For this review, take the finished solid that the model builds, in its own axes (mm). Give positions to 0.01 mm unless a question says otherwise; leave off trailing zeros. Write each loop counter-clockwise with the first axis right and the second up, starting at its lowest first coordinate (ties: lowest second). Pieces come first, ordered by that corner, then holes. Notation, with made-up numbers: (88, 44) -> (111, 44) arc R21 ccw to (111, 56) -> close; hole circle Ø1 at (61.25, 40). An arc over 180 degrees is marked (long way). Return JSON: item names as keys, results as strings.
Autodesk Inventor part; units mm, degrees
ref_plane "YZ Plane" through (0, 0, 0) normal (1, 0, 0) x (0, 1, 0)
ref_plane "XZ Plane" through (0, 0, 0) normal (0, 1, 0) x (-1, 0, 0)
ref_plane "XY Plane" through (0, 0, 0) normal (0, 0, 1) x (1, 0, 0)
sketch "Sketch1" plane through (0, 0, 0) normal (0, 1, 0) x (-1, 0, 0)
  arc A0 (-177, 0) -> (177, 0) centre (0, 0) ccw
  line L0 (-177, 0) -> (-177, 151.6)
  line L1 (-151.6, 177) -> (151.6, 177)
  line L2 (177, 151.6) -> (177, 0)
  arc A1 (-151.6, 177) -> (-177, 151.6) centre (-151.6, 151.6) ccw
  arc A2 (177, 151.6) -> (151.6, 177) centre (151.6, 151.6) ccw
  point P0 (-177, 177)
  point P1 (177, 177)
  dimension "d0" = 354
  dimension "d98" = 177
  dimension "d99" = 177
  dimension "d101" = 354
  dimension "d102" = 177
  dimension "d217" = 25.4
extrude "Extrusion1" add sketch "Sketch1" along normal blind 4.7625
sketch "Sketch8" plane through (0, 4.7625, 0) normal (0, 1, 0) x (1, 0, 0)
  circle A0 centre (101.6, -101.6) radius 1.7
  circle A1 centre (101.6, 101.6) radius 1.7
  circle A2 centre (-101.6, 101.6) radius 1.7
  circle A3 centre (-101.6, -101.6) radius 1.7
  arc A4 (177, 0) -> (-177, 0) centre (0, 0) ccw construction
  line L0 (0, 177) -> (0, -177) construction
  line L1 (-151.6, -177) -> (151.6, -177) construction
  line L2 (-177, 0) -> (-177, -151.6) construction
  line L3 (177, -151.6) -> (177, 0) construction
  line L4 (-177, 0) -> (177, 0) construction
  point P0 (0, 0)
  point P1 (-177, -177)
  point P2 (177, -177)
  dimension "d103" = 3.4
  dimension "d104" = 3.4
  dimension "d105" = 3.4
  dimension "d106" = 3.4
  dimension "d115" = 101.6
  dimension "d116" = 101.6
  dimension "d117" = 101.6
  dimension "d118" = 101.6
  dimension "d119" = 101.6
  dimension "d120" = 101.6
  dimension "d121" = 101.6
  dimension "d122" = 101.6
extrude "Stand-Offs" cut sketch "Sketch8" against normal through all
sketch "Sketch9" plane through (0, 4.7625, 0) normal (0, 1, 0) x (1, 0, 0)
  line L0 (-150.65, -79.3) -> (-150.65, -164.3)
  line L1 (-150.65, -164.3) -> (-120.65, -164.3)
  line L2 (-120.65, -164.3) -> (-120.65, -79.3)
  line L3 (-120.65, -79.3) -> (-150.65, -79.3)
  circle A0 centre (-114.3, -96.4) radius 1.7
  circle A1 centre (-114.3, -147.2) radius 1.7
  circle A2 centre (-157, -147.2) radius 1.7
  circle A3 centre (-157, -96.4) radius 1.7
  arc A4 (177, 0) -> (-177, 0) centre (0, 0) ccw construction
  line L4 (0, 177) -> (0, -177) construction
  line L5 (-151.6, -177) -> (151.6, -177) construction
  line L6 (-177, -177) -> (177, -177) construction
  line L7 (-120.65, -121.8) -> (-150.65, -121.8) construction
  line L8 (150.65, -164.3) -> (120.65, -164.3)
  line L9 (120.65, -164.3) -> (120.65, -79.3)
  line L10 (120.65, -79.3) -> (150.65, -79.3)
  circle A5 centre (114.3, -96.4) radius 1.7
  circle A6 centre (114.3, -147.2) radius 1.7
  line L11 (150.65, -79.3) -> (150.65, -164.3)
  circle A7 centre (157, -96.4) radius 1.7
  circle A8 centre (157, -147.2) radius 1.7
  line L12 (120.65, -121.8) -> (150.65, -121.8) construction
  point P0 (177.1241, 0)
  dimension "d126" = 30
  dimension "d129" = 3.4
  dimension "d130" = 3.4
  dimension "d131" = 3.4
  dimension "d132" = 3.4
  dimension "d133" = 6.35
  dimension "d134" = 6.35
  dimension "d135" = 6.35
  dimension "d136" = 6.35
  dimension "d141" = 120.65
  dimension "d142" = 12.7
  dimension "d143" = 85
  dimension "d144" = 25.4
  dimension "d145" = 25.4
  dimension "d146" = 25.4
  dimension "d147" = 25.4
extrude "Wheels" cut sketch "Sketch9" against normal through all
sketch "Sketch10" plane through (0, 4.7625, 0) normal (0, 1, 0) x (1, 0, 0)
  circle A0 centre (-72.47, -143.49) radius 1.7
  circle A1 centre (-21.59, -143.49) radius 1.7
  circle A2 centre (-72.47, -100.11) radius 1.7
  circle A3 centre (-21.59, -100.11) radius 1.7
  arc A4 (177, 0) -> (-177, 0) centre (0, 0) ccw construction
  line L0 (0, 177) -> (0, -177) construction
  line L1 (-151.6, -177) -> (151.6, -177) construction
  line L2 (177, -151.6) -> (177, 0) construction
  line L3 (-177, 0) -> (-177, -151.6) construction
  line L4 (177, 0) -> (-177, 0) construction
  line L5 (-150.65, -79.3) -> (-150.65, -164.3) construction
  line L6 (-150.65, -121.8) -> (150.65, -121.8) construction
  line L7 (150.65, -79.3) -> (150.65, -164.3) construction
  line L8 (-120.65, -79.3) -> (-120.65, -164.3) construction
  circle A5 centre (72.47, -143.49) radius 1.7
  circle A6 centre (72.47, -100.11) radius 1.7
  circle A7 centre (21.59, -143.49) radius 1.7
  circle A8 centre (21.59, -100.11) radius 1.7
  line L9 (-76.28, -96.3) -> (-17.78, -96.3) construction
  line L10 (-17.78, -96.3) -> (-17.78, -147.3) construction
  line L11 (-17.78, -147.3) -> (-76.28, -147.3) construction
  line L12 (-76.28, -147.3) -> (-76.28, -96.3) construction
  point P0 (-177, -177)
  point P1 (177, -177)
  dimension "d150" = 3.4
  dimension "d151" = 3.4
  dimension "d152" = 3.4
  dimension "d153" = 3.4
  dimension "d235" = 58.5
  dimension "d236" = 51
  dimension "d237" = 3.81
  dimension "d238" = 3.81
  dimension "d239" = 3.81
  dimension "d240" = 3.81
  dimension "d241" = 3.81
  dimension "d242" = 3.81
  dimension "d243" = 3.81
  dimension "d244" = 3.81
  dimension "d245" = 21.59
  dimension "d246" = 21.59
  dimension "d247" = 25.5
extrude "Motor Mount" cut sketch "Sketch10" against normal through all
sketch "Sketch11" plane through (0, 4.7625, 0) normal (0, 1, 0) x (1, 0, 0)
  circle A0 centre (-46.25, 39.25) radius 1.7
  circle A1 centre (46.25, 39.25) radius 1.7
  circle A2 centre (46.25, -39.25) radius 1.7
  circle A3 centre (-46.25, -39.25) radius 1.7
  line L0 (-177, 0) -> (-177, -151.6) construction
  arc A4 (177, 0) -> (-177, 0) centre (0, 0) ccw construction
  line L1 (-177, 0) -> (177, 0) construction
  line L2 (0, 177) -> (0, -177) construction
  line L3 (-151.6, -177) -> (151.6, -177) construction
  point P0 (-177, -177)
  point P1 (177, -177)
  dimension "d170" = 3.4
  dimension "d171" = 3.4
  dimension "d172" = 3.4
  dimension "d173" = 3.4
  dimension "d174" = 92.5
  dimension "d175" = 92.5
  dimension "d176" = 78.5
  dimension "d177" = 78.5
  dimension "d183" = 46.25
  dimension "d184" = 39.25
  dimension "d185" = 39.25
  dimension "d186" = 46.25
extrude "PCB" cut sketch "Sketch11" against normal through all
sketch "Sketch12" plane through (0, 4.7625, 0) normal (0, 1, 0) x (1, 0, 0)
  circle A0 centre (20, 132.55) radius 1.7
  circle A1 centre (-20, 132.55) radius 1.7
  line L0 (-177, 0) -> (-177, -151.6) construction
  arc A2 (177, 0) -> (-177, 0) centre (0, 0) ccw construction
  line L1 (-177, 0) -> (177, 0) construction
  arc A3 (177, 0) -> (-177, 0) centre (0, 0) ccw construction
  line L2 (0, 177) -> (0, -177) construction
  point P0 (-177, -177)
  dimension "d190" = 3.4
  dimension "d191" = 3.4
  dimension "d192" = 40
  dimension "d198" = 44.45
  dimension "d200" = 44.45
  dimension "d201" = 20
extrude "Ball Caster" cut sketch "Sketch12" against normal through all
sketch "Sketch13" plane through (0, 4.7625, 0) normal (0, 1, 0) x (1, 0, 0)
  line L0 (-34.925, 155.575) -> (-28.575, 155.575)
  line L1 (-28.575, 155.575) -> (-28.575, 152.4)
  line L2 (-28.575, 152.4) -> (-34.925, 152.4)
  line L3 (-34.925, 152.4) -> (-34.925, 155.575)
  line L4 (-22.225, 155.575) -> (-15.875, 155.575)
  line L5 (-15.875, 155.575) -> (-15.875, 152.4)
  line L6 (-15.875, 152.4) -> (-22.225, 152.4)
  line L7 (-22.225, 152.4) -> (-22.225, 155.575)
  line L8 (-9.525, 155.575) -> (-3.175, 155.575)
  line L9 (-3.175, 155.575) -> (-3.175, 152.4)
  line L10 (-3.175, 152.4) -> (-9.525, 152.4)
  line L11 (-9.525, 152.4) -> (-9.525, 155.575)
  line L12 (3.175, 155.575) -> (9.525, 155.575)
  line L13 (9.525, 155.575) -> (9.525, 152.4)
  line L14 (9.525, 152.4) -> (3.175, 152.4)
  line L15 (3.175, 152.4) -> (3.175, 155.575)
  line L16 (15.875, 155.575) -> (22.225, 155.575)
  line L17 (22.225, 155.575) -> (22.225, 152.4)
  line L18 (22.225, 152.4) -> (15.875, 152.4)
  line L19 (15.875, 152.4) -> (15.875, 155.575)
  line L20 (28.575, 155.575) -> (34.925, 155.575)
  line L21 (34.925, 155.575) -> (34.925, 152.4)
  line L22 (34.925, 152.4) -> (28.575, 152.4)
  line L23 (28.575, 152.4) -> (28.575, 155.575)
  arc A0 (177, 0) -> (-177, 0) centre (0, 0) ccw construction
  line L24 (0, 177) -> (0, -177) construction
  line L25 (-151.6, -177) -> (151.6, -177) construction
  line L26 (177, -151.6) -> (177, 0) construction
  line L27 (-177, 0) -> (-177, -151.6) construction
  line L28 (177, 0) -> (-177, 0) construction
  point P0 (-177, -177)
  point P1 (177, -177)
  dimension "d204" = 3.175
  dimension "d205" = 6.35
  dimension "d208" = 12.7
  dimension "d213" = 152.4
  dimension "d214" = 3.175
extrude "Switch" cut sketch "Sketch13" against normal through all
equation "\"d101\" = d0"
equation "\"m3_heat_set_insert\" = 4"
equation "\"m3_clearance\" = 3.4"
equation "\"m3_heat_set_depth\" = 7"
equation "\"hardboard_thickness\" = 5"
equation "\"robot_diameter\" = 354"
properties part number "layer1_new_motor2"
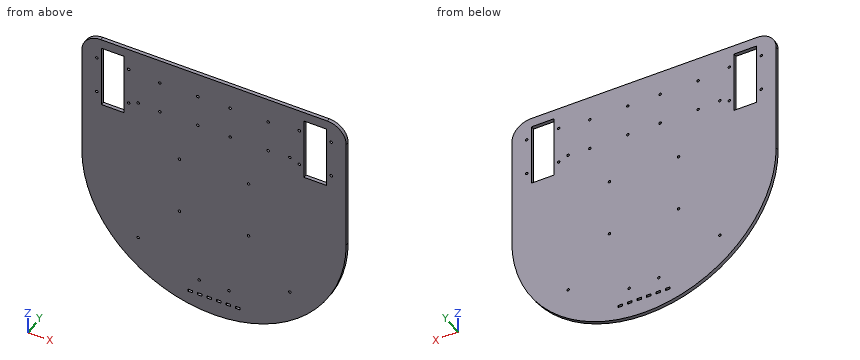
1. For pin 1 (1 mm diameter, centred on y = 3, z = -154.5, fed in from -X); pin 2 (2.5 mm diameter, centred on x = 21.59, z = 143.49, fed in from +Y); pin 3 (1.6 mm diameter, centred on y = 3.5, z = -153.5, fed in from -X); pin 4 (1.4 mm diameter, centred on x = -17.5, y = 2.5, fed in from -Z), all flat-tipped, find the tip position at first contact; note any pin that passes through.
Results found:
{"pin 1": "stops at x = -87.25", "pin 2": "passes through", "pin 3": "stops at x = -89.51", "pin 4": "stops at z = -176.2"}
2. Add section B-B, the plane y = 0.85. Count the separate pieces of the cut face and the enclosed holes in it, plus the area to 3 significant figures.
Results found:
{"separate pieces": "1", "enclosed holes": "34", "area": "106,000 mm²"}
3. Add section C-C, the plane z = -55. State the section outline as (x, y) points, plus the area to 3 significant figures.
Results found:
{"outline": "(-168.24, 0) -> (168.24, 0) -> (168.24, 4.76) -> (-168.24, 4.76) -> close", "area": "1,600 mm²"}
4. To check wall thickness, follow probe 1 along X at (y, z) = (1.65, 116); probe 2 along Z at (x, y) = (46.25, 1.85); probe 3 along Z at (x, y) = (-45, 3.45). State the ranges of each line that lie inside material, in increasing order.
Results found:
{"probe 1": "x = -177 to -150.65, -120.65 to 120.65, 150.65 to 177", "probe 2": "z = -170.85 to -40.95, -37.55 to 37.55, 40.95 to 177", "probe 3": "z = -171.18 to -40.4, -38.1 to 38.1, 40.4 to 177"}
5. Add section A-A, the plane z = 108.5. State the section outline as (x, y) points, plus the area to 3 significant figures.
Results found:
{"outline": "(-177, 0) -> (-150.65, 0) -> (-150.65, 4.76) -> (-177, 4.76) -> close; (-120.65, 0) -> (120.65, 0) -> (120.65, 4.76) -> (-120.65, 4.76) -> close; (150.65, 0) -> (177, 0) -> (177, 4.76) -> (150.65, 4.76) -> close", "area": "1,400 mm²"}
